Autodesk Inventor part; units mm, degrees
ref_plane "YZ Plane" through (0, 0, 0) normal (1, 0, 0) x (0, 1, 0)
ref_plane "XZ Plane" through (0, 0, 0) normal (0, 1, 0) x (-1, 0, 0)
ref_plane "XY Plane" through (0, 0, 0) normal (0, 0, 1) x (1, 0, 0)
sketch "Sketch1" plane through (0, 0, 0) normal (0, 0, 1) x (1, 0, 0)
  line L0 (6.6074, 9.0814) -> (61.6074, 9.0814)
  line L1 (61.6074, 9.0814) -> (61.6074, 16.0814)
  line L2 (52.6074, 19.0814) -> (6.6074, 19.0814)
  line L3 (6.6074, 19.0814) -> (6.6074, 9.0814)
  line L4 (52.6074, 16.0814) -> (52.6074, 19.0814)
  line L5 (52.6074, 16.0814) -> (61.6074, 16.0814)
  dimension "d0" = 55
  dimension "d1" = 7
  dimension "d6" = 9
  dimension "d7" = 3
extrude "Extrusion1" add sketch "Sketch1" along normal blind 70
sketch "Sketch2" plane through (6.6074, 19.0814, 0) normal (0, 1, 0) x (1, 0, 0)
  circle A0 centre (23, -10) radius 4
  circle A1 centre (23, -60) radius 4
  line L0 (46, -70) -> (0, -70)
  line L1 (55, 0) -> (55, -70)
  line L2 (46, 0) -> (0, 0)
  circle A2 centre (30, -35) radius 8
  line L3 (55, 0) -> (55, -70)
  circle A3 centre (50.5, -60) radius 3
  line L4 (46, 0) -> (46, -70)
  line L5 (55, -70) -> (46, -70)
  circle A4 centre (50.5, -41.5) radius 3
  circle A5 centre (50.5, -10) radius 3
  circle A6 centre (50.5, -28.5) radius 3
  line L6 (55, 0) -> (46, 0)
  point P0 (-6.6074, 0)
  dimension "d10" = 8
  dimension "d11" = 8
  dimension "d12" = 10
  dimension "d15" = 10
  dimension "d17" = 16
  dimension "d22" = 6
  dimension "d23" = 4.5
  dimension "d24" = 10
  dimension "d30" = 10
  dimension "d33" = 25
  dimension "d34" = 32
  dimension "d35" = 32
  dimension "d36" = 35
  dimension "d37" = 4.5
  dimension "d38" = 4.5
  dimension "d39" = 4.5
  dimension "d40" = 28.5
  dimension "d41" = 28.5
extrude "Extrusion2" cut sketch "Sketch2" against normal blind 30 contours A0 | A1 | A2 | A3 | A4 | A5 | A6
chamfer "Chaflán1" distance 1 angle 45 1 edges at (52.6074, 19.0814, 35)
equation "\"d24\" = d30"
equation "\"d41\" = d40"
properties part number "Piso, Vínculo Cabezal" material "Aluminum 6061"
Design review of the part built by this model. Coordinates are the model's own, in mm. A direction names the side the tool comes from. Round coordinates to 2 decimals unless told otherwise and drop trailing zeros. Write each loop counter-clockwise with the first axis right and the second up, starting at its lowest first coordinate (ties: lowest second). Pieces come first, ordered by that corner, then holes.
Item 1: We need section D-D on x = 26.5. Write out the cut boundary in (y, z).
Item 2: We need section B-B on z = 10. Write out the cut boundary in (x, y), and give its area (4 significant figures).
Item 3: We need section A-A on z = 35. Write out the cut boundary in (x, y).
Item 4: For probe 1 along X at (y, z) = (13.5, 10); probe 2 along X at (y, z) = (10.5, 28.5); probe 3 along X at (y, z) = (14.25, 34.5), list the stretches that pass through material, from the lowest coordinate up.
Item 5: The part is to be moulded in two halves that separate along X. For faces 3 (the flat face through (52.607, 17, 35)), 4 (the cylindrical face through (54.9, 12.63, 57.97)), 5 (the flat face through (34, 14, 70)), say which applies: +X half, -X half, draft (parallel to the pull), parting line (faces both ways), or undercut.
Item 6: Clearance check with flat-ended pins moving along their axes: pin 1 Ø6.5 at (x, z) = (29.61, 10) entering from -Y; pin 2 Ø9.5 at (x, z) = (57.11, 10) entering from +Y; pin 3 Ø2.5 at (x, z) = (58.5, 17.5) entering from +Y. State where each tip first meets the part, or that it passes through.
Item 7: We need section C-C on y = 11.25. Write out the cut boundary in (x, z).
Item 8: For faces 1 (the flat face through (57, 16.081, 35)), 2 (the cylindrical face through (31.45, 14.15, 63.55)), list the 3-axis set-ups (+Z, -Z, +X, -X, +Y, -Y) from which the entire face can be reached by the end or side of a thin tool; tool diameter is ignored.
Returned:
1. outline: (9.08, 0) - (19.08, 0) - (19.08, 7.48) - (9.08, 7.48) - close; (9.08, 12.52) - (19.08, 12.52) - (19.08, 57.48) - (9.08, 57.48) - close; (9.08, 62.52) - (19.08, 62.52) - (19.08, 70) - (9.08, 70) - close
2. outline: (6.61, 9.08) - (25.61, 9.08) - (25.61, 19.08) - (6.61, 19.08) - close; (33.61, 9.08) - (54.11, 9.08) - (54.11, 16.08) - (52.61, 16.08) - (52.61, 18.08) - (51.61, 19.08) - (33.61, 19.08) - close; (60.11, 9.08) - (61.61, 9.08) - (61.61, 16.08) - (60.11, 16.08) - close
2. area: 400.5 mm2
3. outline: (6.61, 9.08) - (28.61, 9.08) - (28.61, 19.08) - (6.61, 19.08) - close; (44.61, 9.08) - (61.61, 9.08) - (61.61, 16.08) - (52.61, 16.08) - (52.61, 18.08) - (51.61, 19.08) - (44.61, 19.08) - close
4. probe 1: x = 6.61 to 25.61, 33.61 to 54.11, 60.11 to 61.61
4. probe 2: x = 6.61 to 31.94, 41.27 to 54.11, 60.11 to 61.61
4. probe 3: x = 6.61 to 28.62, 44.59 to 61.61
5. face 3: +X half
5. face 4: undercut
5. face 5: draft
6. pin 1: passes through
6. pin 2: stops at y = 18.33
6. pin 3: stops at y = 16.08
7. outline: (6.61, 0) - (61.61, 0) - (61.61, 70) - (6.61, 70) - close; hole circle Ø8 at (29.61, 10); hole circle Ø8 at (29.61, 60); hole circle Ø16 at (36.61, 35); hole circle Ø6 at (57.11, 10); hole circle Ø6 at (57.11, 28.5); hole circle Ø6 at (57.11, 41.5); hole circle Ø6 at (57.11, 60)
8. face 1: +Z, -Z, +X, +Y
8. face 2: +Y, -Y
